Work out the finished part from the listing and answer in its coordinate system (mm). A direction names the side the tool comes from. Coordinates: 2 decimals unless noted, no trailing zeros. Write each loop counter-clockwise with the first axis right and the second up, starting at its lowest first coordinate (ties: lowest second). Pieces come first, ordered by that corner, then holes. Notation, with made-up numbers: (-19.75, -38) - (-3.75, -38) arc R14 ccw to (-3.75, -33) - close; hole circle Ø7 at (-19, 14.25). An arc over 180 degrees is marked (long way). Use a Markdown table: item, result. Add a question column.
(1) Find the intervals of material crossed by line 1 (X direction, y = -305.5, z = 128.5); line 2 (Z direction, x = 57, y = 145), in increasing order. Write a range as from..to.
(2) The part is cut by section B-B, the plane z = 31. Give the vertices of the cut face in (x, y).
(3) For a pull along Z with two mould halves and no side action, classify faces 1 (the face through (-274.53, 89.99, 125.12)), 2 (the face through (-276.5, 5, 70)), 3 (the face through (-4, 5, 0)) as released by +Z, released by -Z, zero draft, split by the parting line, or undercut.
(4) The part is cut by section D-D, the plane z = 156.5. Give the vertices of the cut face in (x, y).
(5) The part is cut by section A-A, the plane y = 21.5. Give the vertices of the cut face in (x, z).
(6) A tool of negligible diameter and unlimited length cuts with its end or side. For faces 4 (the face through (-4, 5, -4)), 5 (the face through (272.5, -5, 73)), 6 (the face through (274.47, -89.99, 126.88)), 7 (the face through (89.99, 200.88, -1.97)), from which of +Z, -Z, +X, -X, +Y, -Y can it reach the whole face along a straight path? Write none if from no direction.
(7) Given pin 1 Ø2 at (x, y) = (130, 224.5) entering from +Z; pin 2 Ø1.2 at (x, y) = (275, 12) entering from -Z, each flat-ended and moving along its own axis, determine where each tip first touches the part or whether it passes through.
(8) The part is cut by section C-C, the plane y = -130. Give the vertices of the cut face in (x, z), then the cut area to 3 significant figures.
from build123d import *

# Parameters (mm, degrees)
SKETCH_1_W                         = 553
SKETCH_1_H                         = 700
SM_BASE_FLANGE_1_DEPTH             = 4
SM_EDGE_FLANGE_1_STRIP_W           = 17.4732
SM_EDGE_FLANGE_1_STRIP_H           = 4
SM_EDGE_FLANGE_1_STRIP_CUT_DEPTH   = 700
SM_EDGE_FLANGE_1_STRIP_2_W         = 17.4732
SM_EDGE_FLANGE_1_STRIP_2_H         = 4
SM_EDGE_FLANGE_1_STRIP_CUT_2_DEPTH = 700
SM_EDGE_FLANGE_1_DEPTH             = 700
SM_EDGE_FLANGE_1_BEND_DEPTH        = 700
CUT_EXTRUDE_1_DEPTH                = 703.741061843
CUT_EXTRUDE_2_DEPTH                = 10
CHAMFER_1_SIZE                     = 5
CUT_EXTRUDE_3_DEPTH                = 703.741061843
PATTERN_LINEAR_1_COUNT             = 6
PATTERN_LINEAR_1_PITCH             = 130


# Sheet-metal steps are written as plain solids
with BuildPart() as part:
    # Sketch 1 → 基体-法兰1 (new body)
    with BuildSketch(Plane.XY):
        Rectangle(SKETCH_1_W, SKETCH_1_H)
    extrude(amount=-SM_BASE_FLANGE_1_DEPTH)

    # 边线-法兰1 strip (across the edge) → 边线-法兰1 strip cut (cut)
    with BuildSketch(Plane(origin=(-276.5, 350, 0), x_dir=(1, 0, 0), z_dir=(0, -1, 0))):
        with Locations((-4, -2)):
            Rectangle(SM_EDGE_FLANGE_1_STRIP_W, SM_EDGE_FLANGE_1_STRIP_H)
    extrude(amount=SM_EDGE_FLANGE_1_STRIP_CUT_DEPTH, mode=Mode.SUBTRACT)

    # 边线-法兰1 strip 2 (across the edge) → 边线-法兰1 strip cut 2 (cut)
    with BuildSketch(Plane(origin=(276.5, -350, 0), x_dir=(-1, 0, 0), z_dir=(0, 1, 0))):
        with Locations((-4, -2)):
            Rectangle(SM_EDGE_FLANGE_1_STRIP_2_W, SM_EDGE_FLANGE_1_STRIP_2_H)
    extrude(amount=SM_EDGE_FLANGE_1_STRIP_CUT_2_DEPTH, mode=Mode.SUBTRACT)

    # 边线-法兰1 section (across the edge) → 边线-法兰1 (add)
    with BuildSketch(Plane(origin=(-276.5, 350, 0), x_dir=(1, 0, 0), z_dir=(0, -1, 0))):
        with BuildLine():
            Line((0, 0.7366), (0, 256))
            Line((0, 256), (4, 256))
            Line((4, 256), (4, 0.7366))
            ThreePointArc((4, 0.7366), (4.215745145, 0.215745145), (4.7366, 0))
            Line((4.7366, 0), (4.7366, -4))
            ThreePointArc((4.7366, -4), (1.38731802, -2.61268198), (0, 0.7366))
        make_face()
    extrude(amount=SM_EDGE_FLANGE_1_DEPTH)

    # 边线-法兰1 section 2 (across the edge) → 边线-法兰1 bend (add)
    with BuildSketch(Plane(origin=(276.5, -350, 0), x_dir=(-1, 0, 0), z_dir=(0, 1, 0))):
        with BuildLine():
            Line((0, 0.7366), (0, 256))
            Line((0, 256), (4, 256))
            Line((4, 256), (4, 0.7366))
            ThreePointArc((4, 0.7366), (4.215745145, 0.215745145), (4.7366, 0))
            Line((4.7366, 0), (4.7366, -4))
            ThreePointArc((4.7366, -4), (1.38731802, -2.61268198), (0, 0.7366))
        make_face()
    extrude(amount=SM_EDGE_FLANGE_1_BEND_DEPTH)

    # 草图15 → 切除-拉伸1 (cut, through all)
    with BuildSketch(Plane.ZY.offset(276.5)):
        with BuildLine():
            Line((166, 50), (166, -50))
            ThreePointArc((166, -50), (126, -90), (86, -50))
            Line((86, -50), (86, 50))
            ThreePointArc((86, 50), (126, 90), (166, 50))
        make_face()
    extrude(amount=-CUT_EXTRUDE_1_DEPTH, mode=Mode.SUBTRACT)

    # 草图16 → 切除-拉伸2 (cut)
    with BuildSketch(Plane.XY):
        with BuildLine():
            Line((-50, 240), (50, 240))
            ThreePointArc((50, 240), (90, 200), (50, 160))
            Line((50, 160), (-50, 160))
            ThreePointArc((-50, 160), (-90, 200), (-50, 240))
        make_face()
    extrude(amount=-CUT_EXTRUDE_2_DEPTH, mode=Mode.SUBTRACT)

    # 倒角1
    chamfer_1_edges = [part.edges().sort_by_distance(p)[0] for p in [
        (-274.5, 350, 256),
        (-274.5, -350, 256),
        (274.5, -350, 256),
        (274.5, 350, 256),
    ]]
    chamfer(chamfer_1_edges, length=CHAMFER_1_SIZE)

    # 草图17 → 切除-拉伸3 (cut, through all)
    with BuildSketch(Plane.ZY.offset(276.5)):
        with BuildLine():
            Line((235.5, 328.5), (241.5, 328.5))
            ThreePointArc((241.5, 328.5), (245, 325), (241.5, 321.5))
            Line((241.5, 321.5), (235.5, 321.5))
            ThreePointArc((235.5, 321.5), (232, 325), (235.5, 328.5))
        make_face()
    cut_extrude_3 = extrude(amount=-CUT_EXTRUDE_3_DEPTH, mode=Mode.SUBTRACT)

    # 阵列(线性)1: 切除-拉伸3 ×6
    with Locations(*[(0, -i * PATTERN_LINEAR_1_PITCH, 0) for i in range(1, PATTERN_LINEAR_1_COUNT)]):
        add(cut_extrude_3, mode=Mode.SUBTRACT)


solid = part.part
Model answer:
| question | item | result |
|---|---|---|
| 1 | line 1 | -276.5..-272.5, 272.5..276.5 |
| 1 | line 2 | -4..0 |
| 2 | outline | (-276.5, -350) - (-272.5, -350) - (-272.5, 350) - (-276.5, 350) - close; (272.5, -350) - (276.5, -350) - (276.5, 350) - (272.5, 350) - close |
| 3 | face 1 | undercut |
| 3 | face 2 | zero draft |
| 3 | face 3 | released by +Z |
| 4 | outline | (-276.5, -350) - (-272.5, -350) - (-272.5, -75.88) - (-276.5, -75.88) - close; (-276.5, 75.88) - (-272.5, 75.88) - (-272.5, 350) - (-276.5, 350) - close; (272.5, -350) - (276.5, -350) - (276.5, -75.88) - (272.5, -75.88) - close; (272.5, 75.88) - (276.5, 75.88) - (276.5, 350) - (272.5, 350) - close |
| 5 | outline | (-276.5, 0.74) arc R4.74 ccw to (-271.76, -4) - (271.76, -4) arc R4.74 ccw to (276.5, 0.74) - (276.5, 86) - (272.5, 86) - (272.5, 0.74) arc R0.74 cw to (271.76, 0) - (-271.76, 0) arc R0.74 cw to (-272.5, 0.74) - (-272.5, 86) - (-276.5, 86) - close; (-276.5, 166) - (-272.5, 166) - (-272.5, 256) - (-276.5, 256) - close; (272.5, 166) - (276.5, 166) - (276.5, 256) - (272.5, 256) - close |
| 6 | face 4 | -Z, +X, -X, +Y, -Y |
| 6 | face 5 | +Z, +Y, -Y |
| 6 | face 6 | +X, -X |
| 6 | face 7 | +Z, -Z |
| 7 | pin 1 | z = 0 |
| 7 | pin 2 | z = -3.2 |
| 8 | outline | (-276.5, 0.74) arc R4.74 ccw to (-271.76, -4) - (271.76, -4) arc R4.74 ccw to (276.5, 0.74) - (276.5, 256) - (272.5, 256) - (272.5, 0.74) arc R0.74 cw to (271.76, 0) - (-271.76, 0) arc R0.74 cw to (-272.5, 0.74) - (-272.5, 256) - (-276.5, 256) - close |
| 8 | area | 4,250 mm^2 |
